Could you check a few things on this model? Use its own coordinates, in mm. A direction names the side the tool comes from. Coordinates: 2 decimals unless noted, no trailing zeros. Order: outer loops, then holes, each group sorted by start corner. A loop starts at its lowest first (then second) coordinate and runs counter-clockwise, first axis right, second up. Notation, with made-up numbers: (-16.5, 11) - (31.5, 11) arc R24 cw to (31.5, 32) - close; hole circle Ø3 at (-11, 25). An arc over 180 degrees is marked (long way). Answer as a JSON object with one key per item and string values. Group by question number.
(1) Imagine slicing it at C-C, the plane z = 1. Write out the boundary of the cut face in (x, y).
(2) Imagine slicing it at D-D, the plane x = -14. Write out the boundary of the cut face in (y, z).
(3) Will these pins go through, and if not, where does the flat tip stop? P1, Ø1.6, axis at x = -12.5, y = -4, coming from the -Z side; P2, Ø4.5, axis at x = 0.5, z = 7.5, coming from the +Y side; P3, Ø5.5, axis at x = 6.5, z = 1.5, coming from the -Y side.
(4) Imagine slicing it at A-A, the plane z = -11.5. Write out the boundary of the cut face in (x, y), and give its area (3 significant figures).
(5) Please list where these lines run through material, in increasing order: probe 1 along Y at (x, z) = (-23, 8.5); probe 2 along Z at (x, y) = (20.5, 3.75); probe 3 along X at (y, z) = (2.25, 13).
(6) Which directions (+Z, -Z, +X, -X, +Y, -Y) give clear straight access to the entire face, cutting with the end or side of a thin tool? Please do faces 1 (the flat face through (1, -4, -4)), 2 (the flat face through (1, -4, -14)), 3 (the flat face through (1, -1, -10)).
(7) Imagine slicing it at B-B, the plane y = 4. Write out the boundary of the cut face in (x, z), and give its area (3 significant figures).
(8) We'd pull the mould along X, two halves only. Please class faces 4 (the flat face through (-1, 5, 30.75)), 5 (the flat face through (1, -5, -9)), 6 (the flat face through (-1, 1, 0)): pulls with the +X half, pulls with the -X half, needs draft (parallel to the pull), parting line crosses it, or undercut.
from build123d import *

# Parameters (mm, degrees)
SKETCH1_W           = 76.2
SKETCH1_H           = 63.5
BOSS_EXTRUDE1_DEPTH = 10
SHELL1_T            = -1
BOSS_EXTRUDE2_DEPTH = 76.2
LPATTERN1_COUNT     = 2
LPATTERN1_PITCH     = 20


with BuildPart() as part:
    # Sketch1 → Boss-Extrude1 (new body)
    with BuildSketch(Plane(origin=(0, 0, 0), x_dir=(1, 0, 0), z_dir=(0, 1, 0))):
        Rectangle(SKETCH1_W, SKETCH1_H)
    extrude(amount=BOSS_EXTRUDE1_DEPTH)

    # Shell1
    shell1_openings = [part.faces().sort_by_distance(p)[0] for p in [
        (0, 10, 0),
    ]]
    offset(amount=SHELL1_T, openings=shell1_openings, kind=Kind.INTERSECTION)

    # Sketch2 → Boss-Extrude2 (add)
    with BuildSketch(Plane(origin=(38.1, 0, 0), x_dir=(0, 0, -1), z_dir=(1, 0, 0))):
        Polygon((10, -3), (14, -3), (14, -5), (4, -5), (4, -3), (8, -3), (8, 0), (10, 0), align=None)
    boss_extrude2 = extrude(amount=-BOSS_EXTRUDE2_DEPTH)

    # LPattern1: Boss-Extrude2 ×2
    with Locations(*[(0, 0, i * LPATTERN1_PITCH) for i in range(1, LPATTERN1_COUNT)]):
        add(boss_extrude2)


solid = part.part
Result set:
{
 "1": {"outline": "(-38.1, 0) - (38.1, 0) - (38.1, 10) - (37.1, 10) - (37.1, 1) - (-37.1, 1) - (-37.1, 10) - (-38.1, 10) - close"},
 "2": {"outline": "(-5, -14) - (-3, -14) - (-3, -10) - (0, -10) - (0, -31.75) - (10, -31.75) - (10, -30.75) - (1, -30.75) - (1, 30.75) - (10, 30.75) - (10, 31.75) - (0, 31.75) - (0, 12) - (-3, 12) - (-3, 16) - (-5, 16) - (-5, 6) - (-3, 6) - (-3, 10) - (0, 10) - (0, -8) - (-3, -8) - (-3, -4) - (-5, -4) - close"},
 "3": {"P1": "stops at z = -14", "P2": "stops at y = 1", "P3": "stops at y = 0"},
 "4": {"outline": "(-38.1, -5) - (38.1, -5) - (38.1, -3) - (-38.1, -3) - close; (-38.1, 0) - (38.1, 0) - (38.1, 10) - (37.1, 10) - (37.1, 1) - (-37.1, 1) - (-37.1, 10) - (-38.1, 10) - close", "area": "247 mm^2"},
 "5": {"probe 1": "y = -5 to -3, 0 to 1", "probe 2": "z = -31.75 to -30.75, 30.75 to 31.75", "probe 3": "x = -38.1 to -37.1, 37.1 to 38.1"},
 "6": {"face 1": "+X, -X, -Y", "face 2": "-Z, +X, -X, -Y", "face 3": "-Z, +X, -X"},
 "7": {"outline": "(-38.1, -31.75) - (38.1, -31.75) - (38.1, 31.75) - (-38.1, 31.75) - close; hole (-37.1, -30.75) - (37.1, -30.75) - (37.1, 30.75) - (-37.1, 30.75) - close", "area": "275 mm^2"},
 "8": {"face 4": "undercut", "face 5": "needs draft", "face 6": "undercut"}
}
